from build123d import *

# Parameters (mm, degrees)
SKETCH1_W             = 76.2
SKETCH1_H             = 78.74
SKETCH1_W_2           = 68.58
SKETCH1_H_2           = 71.12
BOSS_EXTRUDE1_DEPTH   = 50.8
SKETCH1_W_3           = 63.5
SKETCH1_H_3           = 66.04
SKETCH1_W_4           = 58.42
SKETCH1_H_4           = 60.96
BOSS_EXTRUDE1_2_DEPTH = 50.8
SKETCH2_W             = 76.2
SKETCH2_H             = 78.74
SKETCH2_W_2           = 58.42
SKETCH2_H_2           = 60.96
BOSS_EXTRUDE2_DEPTH   = 5.08
SKETCH3_W             = 67.31
SKETCH3_H             = 67.31
SKETCH3_W_2           = 58.42
SKETCH3_H_2           = 60.96
BOSS_EXTRUDE3_DEPTH   = 127


with BuildPart() as part:
    # Sketch1 → Boss-Extrude1 (new body)
    with BuildSketch(Plane.XY):
        with Locations((34.29, 35.56)):
            Rectangle(SKETCH1_W, SKETCH1_H)
        with Locations((34.29, 35.56)):
            Rectangle(SKETCH1_W_2, SKETCH1_H_2, mode=Mode.SUBTRACT)
    extrude(amount=BOSS_EXTRUDE1_DEPTH)



with BuildPart() as body_2:
    # Sketch1 → Boss-Extrude1 2 (new body)
    with BuildSketch(Plane.XY):
        with Locations((34.29, 35.56)):
            Rectangle(SKETCH1_W_3, SKETCH1_H_3)
        with Locations((34.29, 35.56)):
            Rectangle(SKETCH1_W_4, SKETCH1_H_4, mode=Mode.SUBTRACT)
    extrude(amount=BOSS_EXTRUDE1_2_DEPTH)


with BuildPart() as part_1:
    add(part.part)

    add(body_2.part)  # Boss-Extrude2 merges body 2
    # Sketch2 → Boss-Extrude2 (add)
    with BuildSketch(Plane.XY.offset(50.8)):
        with Locations((34.29, 35.56)):
            Rectangle(SKETCH2_W, SKETCH2_H)
        with Locations((34.29, 35.56)):
            Rectangle(SKETCH2_W_2, SKETCH2_H_2, mode=Mode.SUBTRACT)
    extrude(amount=BOSS_EXTRUDE2_DEPTH)

    # Sketch3 → Boss-Extrude3 (add)
    with BuildSketch(Plane.XY.offset(55.88)):
        with Locations((34.29, 35.56)):
            Rectangle(SKETCH3_W, SKETCH3_H)
        with Locations((34.29, 35.56)):
            Rectangle(SKETCH3_W_2, SKETCH3_H_2, mode=Mode.SUBTRACT)
    extrude(amount=BOSS_EXTRUDE3_DEPTH)


solid = part_1.part
Input: part model. Units: mm. Frame: model coordinates. A direction names the side the tool comes from. Give positions to 0.01 mm unless a question says otherwise; leave off trailing zeros. Order: outer loops, then holes, each group sorted by start corner. A loop starts at its lowest first (then second) coordinate and runs counter-clockwise, first axis right, second up. Notation, with made-up numbers: (-16.5, 88) -> (32.5, 88) arc R8 cw to (32.5, 97) -> close; hole circle Ø9 at (-11.75, 35.25). An arc over 180 degrees is marked (long way). Use one line per item in the form item = value.
1) Reachability of faces 5 (the flat face through (0.635, 35, 118)), 6 (the flat face through (5.08, 35, 90)), 7 (the flat face through (67.945, 35, 118)), 8 (the flat face through (0, 35, 25)), 9 (the flat face through (34, 1.905, 118)) from +Z, -Z, +X, -X, +Y, -Y: full face, straight path, thin tool, end or side. Return the list, or none.
Response values:
face_5 = +Z, -X, +Y, -Y
face_6 = +Z, -Z
face_7 = +Z, +X, +Y, -Y
face_8 = -Z
face_9 = +Z, +X, -X, -Y
2) Section C-C, the plane z = 27. Return loops of the section in (x, y), and give its area (3 significant figures).
Response values:
outline = (-3.81, -3.81) -> (72.39, -3.81) -> (72.39, 74.93) -> (-3.81, 74.93) -> close; (2.54, 2.54) -> (66.04, 2.54) -> (66.04, 68.58) -> (2.54, 68.58) -> close; hole (0, 0) -> (68.58, 0) -> (68.58, 71.12) -> (0, 71.12) -> close; hole (5.08, 5.08) -> (63.5, 5.08) -> (63.5, 66.04) -> (5.08, 66.04) -> close
area = 1,750 mm^2
3) First-contact query: pin 1 Ø1.5 at (x, z) = (29, 114) entering from +Y (3 decimals); pin 2 Ø3 at (x, y) = (39.5, 63.5) entering from -Z; pin 3 Ø20 at (y, z) = (50, 91.5) entering from +X (3 decimals); pin 4 Ø12 at (x, z) = (56, 152.5) entering from -Y (3 decimals). Flat tips, straight axial feed; report the tip coordinate or a pass-through.
Response values:
pin_1 = 69.215
pin_2 = through
pin_3 = 67.945
pin_4 = 1.905
4) Mould query, pull axis X, two halves, no side actions, for faces 1 (the flat face through (72.39, 35, 28)), 2 (the flat face through (63.5, 35, 90)), 3 (the flat face through (34, 69.215, 118)), 4 (the flat face through (1, 36, 50.8)). Classes: pulls with the +X half, pulls with the -X half, needs draft (parallel to the pull), parting line crosses it, or undercut.
Response values:
face_1 = pulls with the +X half
face_2 = undercut
face_3 = needs draft
face_4 = undercut
5) Section D-D, the plane x = 43. Return loops of the section in (y, z) (3 decimals).
Response values:
outline = (-3.81, 0) -> (0, 0) -> (0, 50.8) -> (2.54, 50.8) -> (2.54, 0) -> (5.08, 0) -> (5.08, 182.88) -> (1.905, 182.88) -> (1.905, 55.88) -> (-3.81, 55.88) -> close; (66.04, 0) -> (68.58, 0) -> (68.58, 50.8) -> (71.12, 50.8) -> (71.12, 0) -> (74.93, 0) -> (74.93, 55.88) -> (69.215, 55.88) -> (69.215, 182.88) -> (66.04, 182.88) -> close
6) Section A-A, the plane z = 170. Return loops of the section in (x, y) (3 decimals), and give its area (3 significant figures).
Response values:
outline = (0.635, 1.905) -> (67.945, 1.905) -> (67.945, 69.215) -> (0.635, 69.215) -> close; hole (5.08, 5.08) -> (63.5, 5.08) -> (63.5, 66.04) -> (5.08, 66.04) -> close
area = 969 mm^2
7) Line query: probe 1 along X at (y, z) = (56, 10.5); probe 2 along Y at (x, z) = (8, 18.5); probe 3 along X at (y, z) = (9.5, 146) (3 decimals). Output: solid intervals per line, ascending.
Response values:
probe_1 = -3.81 to 0, 2.54 to 5.08, 63.5 to 66.04, 68.58 to 72.39
probe_2 = -3.81 to 0, 2.54 to 5.08, 66.04 to 68.58, 71.12 to 74.93
probe_3 = 0.635 to 5.08, 63.5 to 67.945
8) Section B-B, the plane y = 12. Return loops of the section in (x, z) (3 decimals).
Response values:
outline = (-3.81, 0) -> (0, 0) -> (0, 50.8) -> (2.54, 50.8) -> (2.54, 0) -> (5.08, 0) -> (5.08, 182.88) -> (0.635, 182.88) -> (0.635, 55.88) -> (-3.81, 55.88) -> close; (63.5, 0) -> (66.04, 0) -> (66.04, 50.8) -> (68.58, 50.8) -> (68.58, 0) -> (72.39, 0) -> (72.39, 55.88) -> (67.945, 55.88) -> (67.945, 182.88) -> (63.5, 182.88) -> close
